Could you check a few things on this model? Use its own coordinates, in mm. Face numbers are marked on the shaded views. A direction names the side the tool comes from. Round coordinates to 2 decimals unless told otherwise and drop trailing zeros. Loops run counter-clockwise (first coordinate to the right, second up) from the corner with the lowest first, then second, coordinate; pieces in that order, holes last. Notation, with made-up numbers: (64.25, 12.25) -> (103.25, 12.25) arc R33 cw to (103.25, 47.25) -> close; hole circle Ø4 at (21.5, 34.25). An arc over 180 degrees is marked (long way). One line per item, written item: value.
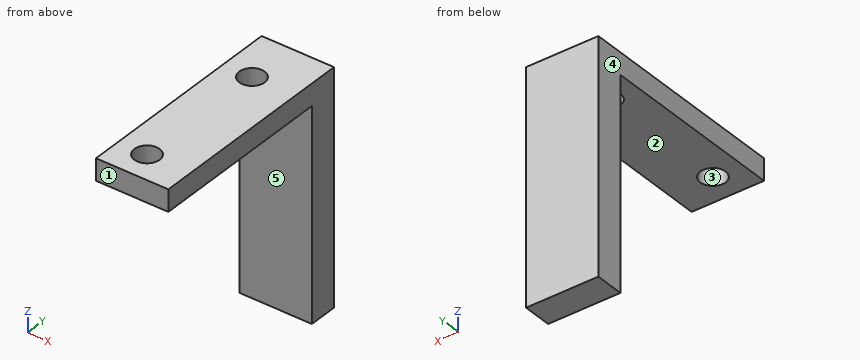
from build123d import *

# Parameters (mm, degrees)
SKETCH1_W           = 10
SKETCH1_H           = 30
SKETCH1_R           = 1.75
BOSS_EXTRUDE1_DEPTH = 32
SKETCH2_W           = 10
SKETCH2_H           = 26
CUT_EXTRUDE1_DEPTH  = 29


with BuildPart() as part:
    # Sketch1 → Boss-Extrude1 (new body)
    with BuildSketch(Plane.XY):
        with Locations((5, -15)):
            Rectangle(SKETCH1_W, SKETCH1_H)
        with Locations((4, -7)):
            Circle(SKETCH1_R, mode=Mode.SUBTRACT)
        with Locations((4, -26)):
            Circle(SKETCH1_R, mode=Mode.SUBTRACT)
    extrude(amount=BOSS_EXTRUDE1_DEPTH)

    # Sketch2 → Cut-Extrude1 (cut)
    with BuildSketch(Plane(origin=(0, 0, 0), x_dir=(-1, 0, 0), z_dir=(0, 0, -1))):
        with Locations((-5, -17)):
            Rectangle(SKETCH2_W, SKETCH2_H)
    extrude(amount=-CUT_EXTRUDE1_DEPTH, mode=Mode.SUBTRACT)


solid = part.part
(1) I'm going to push flat-ended pins straight in: pin 1 Ø1 at (x, z) = (5, 28.5) entering from +Y; pin 2 Ø3 at (x, y) = (7, -12.5) entering from -Z. Where does each tip first touch, or does it pass through?
Recorded:
pin 1: y = 0
pin 2: z = 29
(2) Thinking about a two-plate mould opening in X: for the marked faces 3, 4 and 5, which applies, released by +X, released by -X, zero draft, split by the parting line, or undercut?
Recorded:
face 3: undercut
face 4: released by -X
face 5: zero draft
(3) If we section it at D-D, the plane z = 19: Please give me the cut outline in (x, y), then the cut area to 3 significant figures.
Recorded:
outline: (0, -4) -> (10, -4) -> (10, 0) -> (0, 0) -> close
area: 40.0 mm²
(4) If we section it at C-C, the plane x = 6.25: Please give me the cut outline in (y, z), then the cut area to 3 significant figures.
Recorded:
outline: (-30, 29) -> (-4, 29) -> (-4, 0) -> (0, 0) -> (0, 32) -> (-30, 32) -> close
area: 206 mm²
(5) If I drill on L1, parallel to Y at x = 4, z = 30.8; L2, parallel to X at y = -7, z = 31.15; L3, parallel to Y at x = 9.75, z = 18.5, over which ranges is the centre line in solid material (lowest first)?
Recorded:
L1: -30 to -27.75, -24.25 to -8.75, -5.25 to 0
L2: 0 to 2.25, 5.75 to 10
L3: -4 to 0
(6) If we section it at B-B, the plane x = 4: Please give me the cut outline in (y, z), then the cut area to 3 significant figures.
Recorded:
outline: (-30, 29) -> (-27.75, 29) -> (-27.75, 32) -> (-30, 32) -> close; (-24.25, 29) -> (-8.75, 29) -> (-8.75, 32) -> (-24.25, 32) -> close; (-5.25, 29) -> (-4, 29) -> (-4, 0) -> (0, 0) -> (0, 32) -> (-5.25, 32) -> close
area: 185 mm²
(7) If we section it at A-A, the plane y = -26: Please give me the cut outline in (x, z), then the cut area to 3 significant figures.
Recorded:
outline: (0, 29) -> (2.25, 29) -> (2.25, 32) -> (0, 32) -> close; (5.75, 29) -> (10, 29) -> (10, 32) -> (5.75, 32) -> close
area: 19.5 mm²
(8) For the marked faces 1 and 2, which set-ups out of +Z, -Z, +X, -X, +Y, -Y let a thin tool reach every point of the face, with its end or its side?
Recorded:
face 1: +Z, -Z, +X, -X, -Y
face 2: -Z, +X, -X, -Y
